```python
from build123d import *

# Parameters (mm, degrees)
SKETCH3_R           = 11.1
SKETCH3_R_2         = 5.1
SKETCH3_R_3         = 1.5
BOSS_EXTRUDE5_DEPTH = 4
SKETCH16_R          = 5.1
BOSS_EXTRUDE6_DEPTH = 30
SKETCH17_R          = 11.1
BOSS_EXTRUDE8_DEPTH = 5
SKETCH19_R          = 1


with BuildPart() as part:
    # Sketch3 → Boss-Extrude5 (new body)
    with BuildSketch(Plane.XY):
        Circle(SKETCH3_R)
        Circle(SKETCH3_R_2, mode=Mode.SUBTRACT)
        with Locations((0, 8)):
            Circle(SKETCH3_R_3, mode=Mode.SUBTRACT)
        with Locations((8, 0)):
            Circle(SKETCH3_R_3, mode=Mode.SUBTRACT)
        with Locations((0, -8)):
            Circle(SKETCH3_R_3, mode=Mode.SUBTRACT)
        with Locations((-8, 0)):
            Circle(SKETCH3_R_3, mode=Mode.SUBTRACT)
    extrude(amount=BOSS_EXTRUDE5_DEPTH)

    # Sketch16 → Boss-Extrude6 (add)
    with BuildSketch(Plane(origin=(0, 0, 0), x_dir=(-1, 0, 0), z_dir=(0, 0, -1))):
        Circle(SKETCH16_R)
    extrude(amount=-BOSS_EXTRUDE6_DEPTH)

    # Sketch17 → Boss-Extrude8 (add)
    with BuildSketch(Plane.XY.offset(30)):
        Circle(SKETCH17_R)
    extrude(amount=BOSS_EXTRUDE8_DEPTH)

    # Sweep1: sweep along a path in Sketch20
    with BuildLine(Plane(origin=(0, 0, 0), x_dir=(0, 0, -1), z_dir=(1, 0, 0))) as sweep1_path:
        Line((-30, 9.6), (-12.990250678, 3.71200985))
    # Sketch19 → Sweep1 (sweep)
    with BuildSketch(Plane(origin=(0, 0, 30), x_dir=(-1, 0, 0), z_dir=(0, 0, -1))):
        with Locations((0, 9.6)):
            Circle(SKETCH19_R)
    sweep(path=sweep1_path.line)


solid = part.part
```
The listing builds one solid part. Answer for the finished solid, in the listing's coordinates (mm). A direction names the side the tool comes from. Coordinates: 2 decimals unless noted, no trailing zeros. Write each loop counter-clockwise with the first axis right and the second up, starting at its lowest first coordinate (ties: lowest second). Pieces come first, ordered by that corner, then holes. Notation, with made-up numbers: (27.5, 0) -> (38.5, 0) arc R6 cw to (38.5, 6) -> close; hole circle Ø8 at (-38, -33). An arc over 180 degrees is marked (long way). Write each question's results on one line, items separated by ' | '. Start each with the question number.
1) For a pull along X with two mould halves and no side action, classify faces 1 (the flat face through (0, 0, 0)), 2 (the cylindrical face through (5.97, 9.36, 1.97)), 3 (the cylindrical face through (-0.325, 6.536, 1.972)), 4 (the cylindrical face through (-0.325, -9.464, 1.972)) as +X half, -X half, draft (parallel to the pull), parting line (faces both ways), or undercut.
2) Straight lines are drawn through the part: probe 1 along Y at (x, z) = (0, 3); probe 2 along Z at (x, y) = (10.25, -2.25); probe 3 along Y at (x, z) = (-0.75, 2). For each, find the intervals that lie inside material, in ascending order.
3) A cutting plane is placed at B-B (y = -8.5). Determine the outline of the cut face in (x, z), then the cut area to 3 significant figures.
4) A cutting plane is placed at A-A (x = 8). Determine the outline of the cut face in (y, z), then the cut area to 3 significant figures.
5) A cutting plane is placed at D-D (x = 0). Count the separate pieces of the cut face and the enclosed holes in it, then the cut area to 3 significant figures.
6) A tool of negligible diameter and unlimited length cuts with its end or side. For faces 5 (the cylindrical face through (-2.4, -4.5, 16.8)), 6 (the cylindrical face through (6.5, 0.07, 1.97)), 7 (the flat face through (0, 0, 35)), from which of +Z, -Z, +X, -X, +Y, -Y can it reach the whole face along a straight path? Write none if from no direction.
7) A cutting plane is placed at C-C (z = 2). Determine the outline of the cut face in (x, y), then the cut area to 3 significant figures.
8) Flat-ended cylindrical pins translate along their axes: pin 1 Ø4 at (x, z) = (6, 27.5) entering from +Y; pin 2 Ø5 at (x, y) = (8, 0) entering from -Z; pin 3 Ø5 at (x, z) = (-6, 8.5) entering from +Y; pin 4 Ø2.5 at (x, y) = (0, -8) entering from -Z. Find the tip coordinate at first contact, or state that the pin passes through.
Values follow:
1) face 1: draft | face 2: parting line | face 3: undercut | face 4: undercut
2) probe 1: -11.1 to -9.5, -6.5 to 6.5, 9.5 to 11.1 | probe 2: 0 to 4, 30 to 35 | probe 3: -11.07 to -9.3, -6.7 to 6.7, 9.3 to 11.07
3) outline: (-7.14, 0) -> (-1.41, 0) -> (-1.41, 4) -> (-7.14, 4) -> close; (-7.14, 30) -> (7.14, 30) -> (7.14, 35) -> (-7.14, 35) -> close; (1.41, 0) -> (7.14, 0) -> (7.14, 4) -> (1.41, 4) -> close | area: 117 mm²
4) outline: (-7.69, 0) -> (-1.5, 0) -> (-1.5, 4) -> (-7.69, 4) -> close; (-7.69, 30) -> (7.69, 30) -> (7.69, 35) -> (-7.69, 35) -> close; (1.5, 0) -> (7.69, 0) -> (7.69, 4) -> (1.5, 4) -> close | area: 127 mm²
5) separate pieces: 3 | enclosed holes: 1 | area: 467 mm²
6) face 5: none | face 6: -Z | face 7: +Z, +X, -X, +Y, -Y
7) outline: circle Ø22.2 at (0, 0); hole circle Ø3 at (-8, 0); hole circle Ø3 at (0, -8); hole circle Ø3 at (0, 8); hole circle Ø3 at (8, 0) | area: 359 mm²
8) pin 1: y = 3.16 | pin 2: z = 0 | pin 3: y = 3.71 | pin 4: z = 30
